Study the drawing (mm; zero at the part's minimum x, y, z) and answer. Coordinates: 2 decimals unless noted, no trailing zeros. Loops run counter-clockwise (first coordinate to the right, second up) from the corner with the lowest first, then second, coordinate; pieces in that order, holes last. Notation, with made-up numbers: (56, 0) - (75, 0) arc R22 cw to (75, 38) - close; hole circle Ø8 at (69, 62.25). An arc over 180 degrees is marked (long way). Use one line per item in the form item = value. Start each with the question number.
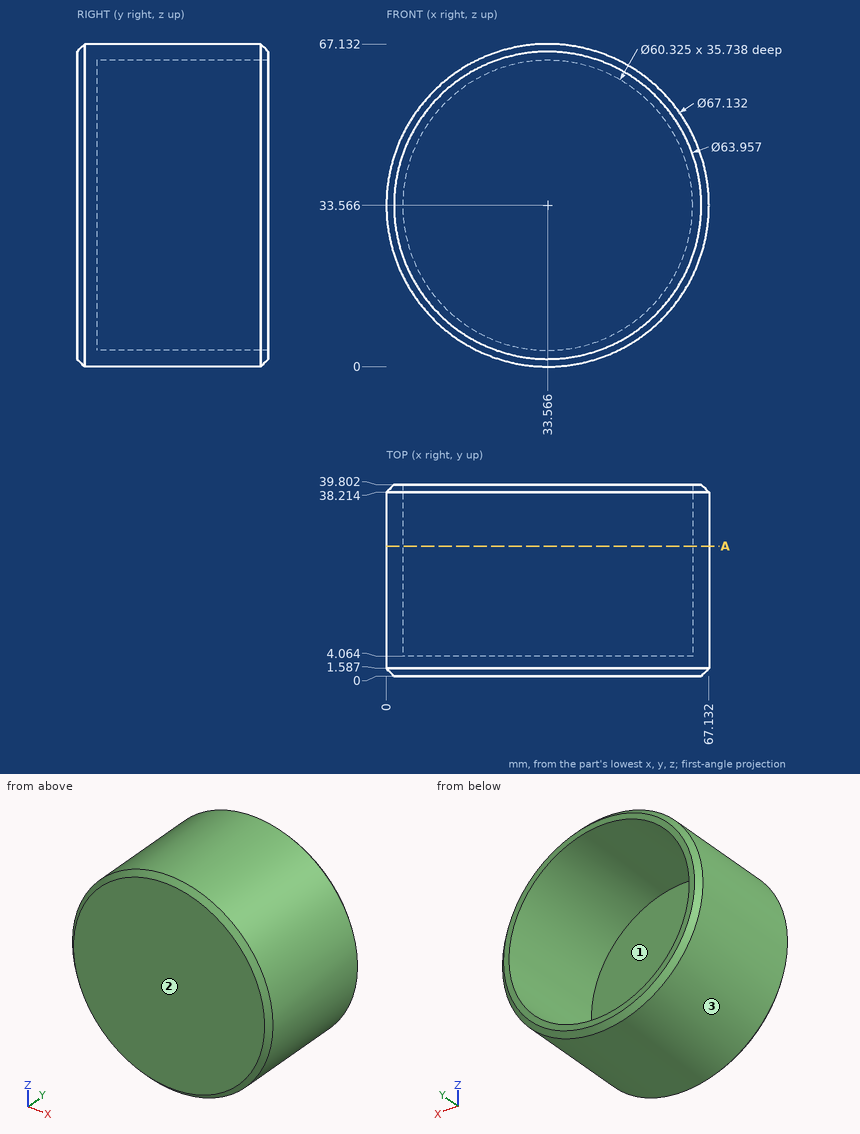
(1) Each of these flat-tipped pins is pushed along its axis until it touches: pin 1 Ø3 at (y, z) = (16, 60) entering from +X; pin 2 Ø3 at (y, z) = (22.5, 46) entering from +X; pin 3 Ø2 at (x, y) = (55.5, 13.5) entering from +Z (1 decimal). Where does it stop, or does it pass through?
(2) Determine the mould class of the marked faces 1, 2 and 3 for opening direction X: +X half, -X half, draft (parallel to the pull), parting line (faces both ways), or undercut.
(3) Find the intervals of material crossed by probe 1 along Z at (x, y) = (34.5, 5.5) (1 decimal); probe 2 along Y at (x, z) = (17, 57) (1 decimal); probe 3 along Z at (x, y) = (33.5, 3.5), in increasing order. Write a range as from..to.
(4) A cutting plane is placed at A-A (y = 27). Determine the outline of the cut face in (x, z) (1 decimal).
Evaluation:
q1.pin_1 = 56.04
q1.pin_2 = 65.3
q1.pin_3 = 59.8
q2.face_1 = undercut
q2.face_2 = draft
q2.face_3 = parting line
q3.probe_1 = 0..3.4, 63.7..67.1
q3.probe_2 = 0..4.1
q3.probe_3 = 0..67.13
q4.outline = circle Ø67.1 at (33.6, 33.6); hole circle Ø60.3 at (33.6, 33.6)
